```python
from build123d import *

# Parameters (mm, degrees)
F0_W     = 406.4
F0_H     = 505
F1_DEPTH = 3
F3_D     = 6.6
F4_DEPTH = 25
F5_W     = 25
F5_H     = 3
F6_DEPTH = 25


with BuildPart() as f1:
    # F0 (on Top) → F1 (new body)
    with BuildSketch(Plane.XY):
        with Locations((-38.4776114106, 56.445750549)):
            Rectangle(F0_W, F0_H)
    extrude(amount=F1_DEPTH)

    # F3 (through all)
    with Locations(Plane.XY.offset(3)):
        with Locations((-114.6776114106, 181.945750549), (37.7223885894, 181.945750549), (37.7223885894, -72.054249451), (-114.6776114106, -72.054249451)):
            Hole(F3_D / 2)

    # F2 (on face) → F4 (cut)
    with BuildSketch(Plane.XY.offset(3)):
        with BuildLine():
            Line((12.3223885894, 181.945750549), (-89.2776114106, 181.945750549))
            ThreePointArc((-89.2776114106, 181.945750549), (-107.2381236528, 174.5062627912), (-114.6776114106, 156.545750549))
            Line((-114.6776114106, 156.545750549), (-114.6776114106, -46.654249451))
            ThreePointArc((-114.6776114106, -46.654249451), (-107.2381236528, -64.6147616931), (-89.2776114106, -72.054249451))
            Line((-89.2776114106, -72.054249451), (12.3223885894, -72.054249451))
            ThreePointArc((12.3223885894, -72.054249451), (30.2829008315, -64.6147616931), (37.7223885894, -46.654249451))
            Line((37.7223885894, -46.654249451), (37.7223885894, 156.545750549))
            ThreePointArc((37.7223885894, 156.545750549), (30.2829008315, 174.5062627912), (12.3223885894, 181.945750549))
        make_face()
    extrude(amount=-F4_DEPTH, mode=Mode.SUBTRACT)

    # F5 (on face) → F6 (cut)
    with BuildSketch(Plane.XY.offset(3)):
        with Locations((-179.1776114106, 282.445750549)):
            Rectangle(F5_W, F5_H)
        with Locations((102.2223885894, 282.445750549)):
            Rectangle(F5_W, F5_H)
        with Locations((102.2223885894, -169.554249451)):
            Rectangle(F5_W, F5_H)
        with Locations((-179.1776114106, -169.554249451)):
            Rectangle(F5_W, F5_H)
    extrude(amount=-F6_DEPTH, mode=Mode.SUBTRACT)


solid = f1.part
```
Can you work these out from the model? Positions are in its coordinate system, mm. A direction names the side the tool comes from. Coordinates: 2 decimals unless noted, no trailing zeros. Order: outer loops, then holes, each group sorted by start corner. A loop starts at its lowest first (then second) coordinate and runs counter-clockwise, first axis right, second up. Notation, with made-up numbers: (73.5, 50.5) - (89.5, 50.5) arc R13 ccw to (89.5, 68.5) - close; hole circle Ø7 at (42.25, 25). An arc over 180 degrees is marked (long way). Answer in a Markdown table with one row per item.
1. If I drill on line 1 along Y through (x, z) = (-187, 2); line 2 along Y through (x, z) = (-4, 1.8); line 3 along X through (y, z) = (4, 0.2), over which ranges is the centre line in solid material (lowest first)?
Reply:
| item | result |
|---|---|
| line 1 | y = -196.05 to -171.05, -168.05 to 280.95, 283.95 to 308.95 |
| line 2 | y = -196.05 to -72.05, 181.95 to 308.95 |
| line 3 | x = -241.68 to -114.68, 37.72 to 164.72 |
2. For pin 1 (1 mm diameter, centred on x = -62, y = -132.5, fed in from -Z), with a flat end and sliding along its axis, tell me the tip position at first contact or that it passes through.
Reply:
| item | result |
|---|---|
| pin 1 | stops at z = 0 |
3. Suppose I cut it at B-B (z = 0.85). Give the number of separate pieces and of enclosed holes in the cut face, and give its area (3 significant figures).
Reply:
| item | result |
|---|---|
| separate pieces | 1 |
| enclosed holes | 9 |
| area | 167,000 mm^2 |
4. If we mould it in two halves opening along X, with no side actions, what happens to faces 3 (the cylindrical face through (30.084, -64.811, 1.521)), 4 (the flat face through (49, 60, 3))? For each: pulls with the +X half, pulls with the -X half, needs draft (parallel to the pull), parting line crosses it, or undercut.
Reply:
| item | result |
|---|---|
| face 3 | undercut |
| face 4 | needs draft |
5. Suppose I cut it at A-A (y = 73.5). Please give me the cut outline in (x, z), and give its area (3 significant figures).
Reply:
| item | result |
|---|---|
| outline | (-241.68, 0) - (-114.68, 0) - (-114.68, 3) - (-241.68, 3) - close; (37.72, 0) - (164.72, 0) - (164.72, 3) - (37.72, 3) - close |
| area | 762 mm^2 |
6. For faces 1 (the cylindrical face through (-107.04, 174.7, 1.52)), 2 (the flat face through (49, 60, 0)), which set-ups out of +Z, -Z, +X, -X, +Y, -Y let a thin tool reach every point of the face, with its end or its side?
Reply:
| item | result |
|---|---|
| face 1 | +Z, -Z |
| face 2 | -Z, +X, -X, +Y, -Y |
